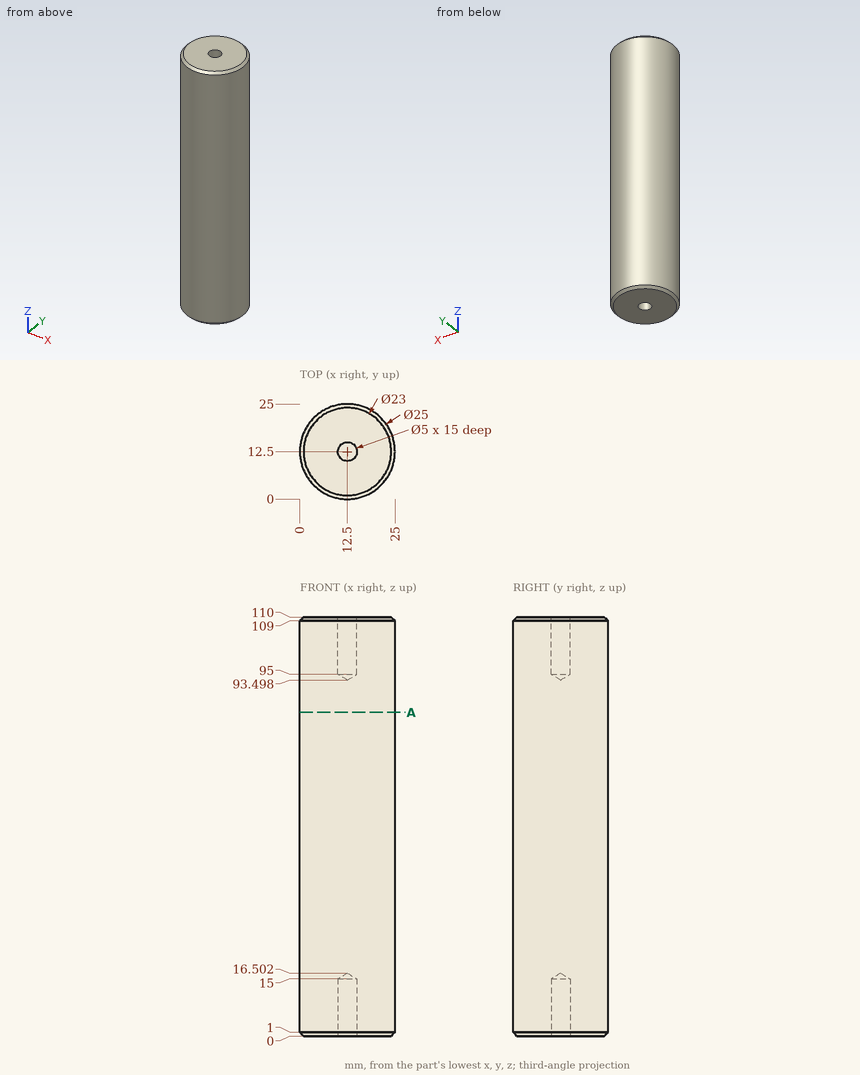
For this review, use the dimensioned drawing (mm, ordinates from the lowest corner) and the shaded views. Give positions to 0.01 mm unless a question says otherwise; leave off trailing zeros. Loops run counter-clockwise (first coordinate to the right, second up) from the corner with the lowest first, then second, coordinate; pieces in that order, holes last.
Item 1: For line 1 along Y through (x, z) = (12.5, 7.25); line 2 along Y through (x, z) = (12, 77.5); line 3 along Y through (x, z) = (5.5, 54), list the stretches that pass through material, from the lowest coordinate up.
Item 2: Insertion check: pin 1 (3 mm diameter, centred on y = 11.5, z = 53.5, fed in from +X); pin 2 (1.5 mm diameter, centred on y = 3.5, z = 88.5, fed in from +X); pin 3 (4 mm diameter, centred on x = 12.5, y = 12.5, fed in from -Z). Each pin has a flat end and moves straight along its axis. Give the tip position at first contact, or say it passes through.
Item 3: Take a section at A-A, the plane z = 85. State the section outline as (x, y) points.
Calculated:
1. line 1: y = 0 to 10, 15 to 25
1. line 2: y = 0.01 to 24.99
1. line 3: y = 2.14 to 22.86
2. pin 1: stops at x = 25
2. pin 2: stops at x = 21.89
2. pin 3: stops at z = 15.3
3. outline: circle Ø25 at (12.5, 12.5)
